Job drawing, mm, ordinate dimensions from the low corner. One solid piece. Coordinates: 2 decimals unless noted, no trailing zeros. Write each loop counter-clockwise with the first axis right and the second up, starting at its lowest first coordinate (ties: lowest second). Pieces come first, ordered by that corner, then holes.
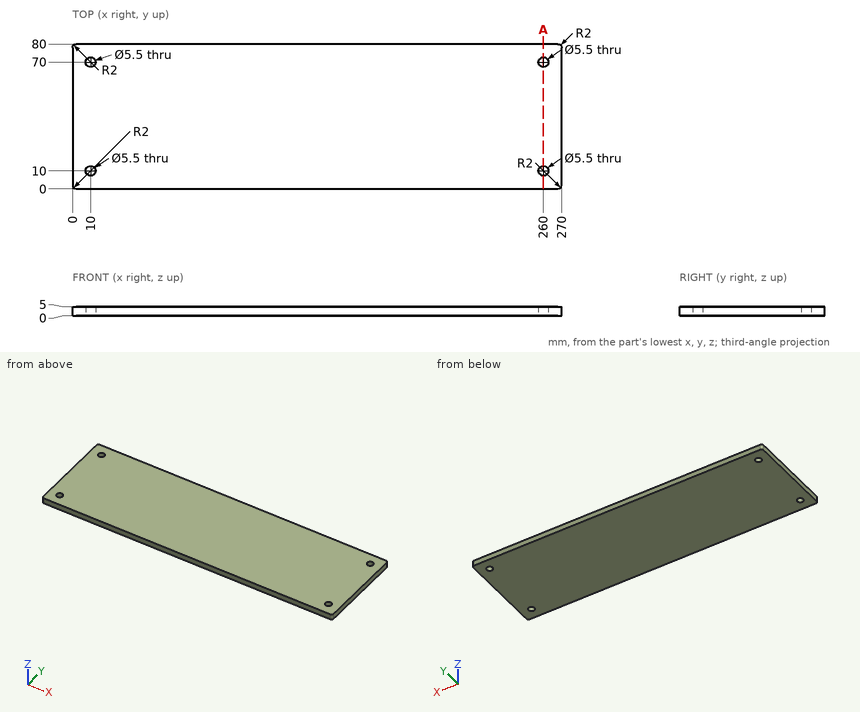
1. Flat gauge pin, fed straight in: pin 1 (4.5 mm diameter, centred on x = 10, y = 70, fed in from -Z). Where does the tip first touch, or does it go through?
Computed values:
pin 1: passes through
2. Saw through at A-A on x = 260. List the corners of the cut face in (y, z), plus the area to 3 significant figures.
Computed values:
outline: (0, 0) - (7.25, 0) - (7.25, 5) - (0, 5) - close; (12.75, 0) - (67.25, 0) - (67.25, 5) - (12.75, 5) - close; (72.75, 0) - (80, 0) - (80, 5) - (72.75, 5) - close
area: 345 mm2
3. Probe line 1 along Y through (x, z) = (260, 3.7); line 2 along X through (y, z) = (10, 1.7). List the from-to ranges inside material, lowest first.
Computed values:
line 1: y = 0 to 7.25, 12.75 to 67.25, 72.75 to 80
line 2: x = 0 to 7.25, 12.75 to 257.25, 262.75 to 270
